Geometry check sheet. Reference: the model listing, model coordinates, mm. A direction names the side the tool comes from. Coordinates: 2 decimals unless noted, no trailing zeros. Write each loop counter-clockwise with the first axis right and the second up, starting at its lowest first coordinate (ties: lowest second). Pieces come first, ordered by that corner, then holes.
from build123d import *

# Parameters (mm, degrees)
F0_R      = 16.129
F1_DEPTH  = 12.7
F2_R      = 22.479
F2_R_2    = 16.129
F3_DEPTH  = 12.7
F5_D      = 3.2639
F5_DEPTH  = 19.05
F5_TIP    = 0.9805744872
F7_DEPTH  = 12.7
F8_R      = 12.7
F9_R      = 7.366
F10_DEPTH = 152.4
F11_R     = 1.27
F13_D     = 3.175
F13_DEPTH = 12.7
F13_TIP   = 0.9538662327
F15_D     = 4.7625
F15_DEPTH = 19.05
F15_TIP   = 1.4307993491
F16_W     = 25.4
F16_H     = 25.5016
F17_DEPTH = 4.7625


with BuildPart() as f1:
    # F0 (on Top) → F1 (new body)
    with BuildSketch(Plane.XY):
        with BuildLine():
            Line((0, 133.35), (0, 0))
            Line((0, 0), (95.25, 0))
            ThreePointArc((95.25, 0), (99.7401280605, 1.8598719395), (101.6, 6.35))
            Line((101.6, 6.35), (101.6, 133.35))
            ThreePointArc((101.6, 133.35), (99.7401280605, 137.8401280605), (95.25, 139.7))
            Line((95.25, 139.7), (6.35, 139.7))
            ThreePointArc((6.35, 139.7), (1.8598719395, 137.8401280605), (0, 133.35))
        make_face()
        with Locations((25.4, 53.975)):
            Circle(F0_R, mode=Mode.SUBTRACT)
    extrude(amount=F1_DEPTH)

    # F2 (on face) → F3 (join)
    with BuildSketch(Plane.XY.offset(12.7)):
        with Locations((25.4, 53.975)):
            Circle(F2_R)
        with Locations((25.4, 53.975)):
            Circle(F2_R_2, mode=Mode.SUBTRACT)
    extrude(amount=F3_DEPTH)

    # F5
    with Locations(Plane.XY.offset(12.7)):
        with Locations((88.265, 127), (88.265, 114.3)):
            Hole(F5_D / 2, depth=F5_DEPTH)
            with Locations((0, 0, -(F5_DEPTH + F5_TIP / 2))):  # 118° drill point
                Cone(0, F5_D / 2, F5_TIP, mode=Mode.SUBTRACT)

    # F6 (on face) → F7 (cut, through all)
    with BuildSketch(Plane.XY.offset(12.7)):
        Polygon((95.25, 0), (0, 28.575), (0, 0), align=None)
        Polygon((0, 139.7), (0, 76.2), (69.85, 139.7), align=None)
    extrude(amount=-F7_DEPTH, mode=Mode.SUBTRACT)

    # F8
    f8_edges = [f1.edges().sort_by_distance(p)[0] for p in [
        (0, 28.575, 6.35),
        (0, 76.2, 6.35),
        (69.85, 139.7, 6.35),
        (95.25, 0, 6.35),
    ]]
    fillet(f8_edges, radius=F8_R)

    # F9 (on Front) → F10 (cut)
    with BuildSketch(Plane.XZ):
        with Locations((76.2, 15.875)):
            Circle(F9_R)
    extrude(amount=-F10_DEPTH, mode=Mode.SUBTRACT)

    # F11
    f11_edges = [f1.edges().sort_by_distance(p)[0] for p in [
        (2.921, 53.975, 25.4),
    ]]
    fillet(f11_edges, radius=F11_R)

    # F13
    with Locations(Plane(origin=(0, 0, 0), x_dir=(0, 1, 0), z_dir=(-1, 0, 0))):
        with Locations((53.975, -18.3411143556)):
            Hole(F13_D / 2, depth=F13_DEPTH)
            with Locations((0, 0, -(F13_DEPTH + F13_TIP / 2))):  # 118° drill point
                Cone(0, F13_D / 2, F13_TIP, mode=Mode.SUBTRACT)

    # F15
    with Locations(Plane.XY.offset(12.7)):
        with Locations((88.9, 101.6), (88.9, 88.9), (63.5, 101.6), (63.5, 88.9), (63.5, 31.75), (63.5, 19.05), (88.9, 19.05), (88.9, 31.75)):
            Hole(F15_D / 2, depth=F15_DEPTH)
            with Locations((0, 0, -(F15_DEPTH + F15_TIP / 2))):  # 118° drill point
                Cone(0, F15_D / 2, F15_TIP, mode=Mode.SUBTRACT)

    # F16 (on face) → F17 (cut)
    with BuildSketch(Plane(origin=(0, 0, 0), x_dir=(1, 0, 0), z_dir=(0, 0, -1))):
        with Locations((88.9, -120.5992)):
            Rectangle(F16_W, F16_H)
    extrude(amount=-F17_DEPTH, mode=Mode.SUBTRACT)


solid = f1.part
1. Draft check along X on faces 4 (the flat face through (22, 70, 25.4)), 5 (the flat face through (47.68, 14.27, 6.44)), 6 (the cylindrical face through (87.62, 90.91, 6.26)). Enter one of: released by +X, released by -X, zero draft, split by the parting line, or undercut.
Computed values:
face 4: zero draft
face 5: released by -X
face 6: undercut
2. Gauge pin test, flat ends, axial feed: pin 1 Ø5.5 at (x, y) = (90.5, 49) entering from +Z; pin 2 Ø2.5 at (y, z) = (53.98, 18.34) entering from -X; pin 3 Ø4 at (x, z) = (91.5, 3.5) entering from -Y. Record the tip position at first contact, or that the pin passes through.
Computed values:
pin 1: stops at z = 12.7
pin 2: stops at x = 41.48
pin 3: stops at y = 2.48
3. Sectioned sample at B-B, the plane x = 25.4. Record the boundary of the cut face in (y, z) (3 decimals), and give its area (3 significant figures).
Computed values:
outline: (20.955, 0) - (37.846, 0) - (37.846, 25.4) - (32.766, 25.4) arc R1.27 ccw to (31.496, 24.13) - (31.496, 12.7) - (20.955, 12.7) - close; (70.104, 0) - (99.291, 0) - (99.291, 12.7) - (76.454, 12.7) - (76.454, 24.13) arc R1.27 ccw to (75.184, 25.4) - (70.104, 25.4) - close
area: 746 mm2
4. Sectioned sample at D-D, the plane y = 123. Record the boundary of the cut face in (x, z) (1 decimal), and give its area (3 significant figures).
Computed values:
outline: (51.5, 0) - (76.2, 0) - (76.2, 4.8) - (101.6, 4.8) - (101.6, 12.7) - (82.8, 12.7) arc R7.4 cw to (69.6, 12.7) - (51.5, 12.7) - close
area: 476 mm2
5. Access from +Z, -Z, +X, -X, +Y, -Y to the whole of each face (thin tool, end or side, straight path). Record for faces 1 (the flat face through (89, 133.35, 2)), 2 (the flat face through (92, 72, 12.7)), 3 (the cylindrical face through (63.81, 103.96, 6.26)).
Computed values:
face 1: -Z, +X
face 2: +Z, +X, +Y, -Y
face 3: +Z, -Z
6. Sectioned sample at A-A, the plane y = 88.9. Record the boundary of the cut face in (x, z) (3 decimals), and give its area (3 significant figures).
Computed values:
outline: (13.97, 0) - (61.119, 0) - (61.119, 12.7) - (13.97, 12.7) - close; (65.881, 0) - (86.519, 0) - (86.519, 12.7) - (82.847, 12.7) arc R7.366 cw to (69.553, 12.7) - (65.881, 12.7) - close; (91.281, 0) - (101.6, 0) - (101.6, 12.7) - (91.281, 12.7) - close
area: 952 mm2
7. Thickness scan on line 1 along Y through (x, z) = (63.5, 4.25) (3 decimals); line 2 along Y through (x, z) = (35.5, 6.75) (3 decimals); line 3 along Z through (x, y) = (50, 60). Record the ranges inside material, lowest first.
Computed values:
line 1: y = 9.525 to 16.669, 21.431 to 29.369, 34.131 to 86.519, 91.281 to 99.219, 103.981 to 133.927
line 2: y = 17.925 to 41.4, 66.55 to 108.473
line 3: z = 0 to 12.7
8. Sectioned sample at C-C, the plane x = 63.5. Record the boundary of the cut face in (y, z) (3 decimals).
Computed values:
outline: (9.525, 0) - (16.669, 0) - (16.669, 12.7) - (9.525, 12.7) - close; (21.431, 0) - (29.369, 0) - (29.369, 12.7) - (21.431, 12.7) - close; (34.131, 0) - (86.519, 0) - (86.519, 12.7) - (34.131, 12.7) - close; (91.281, 0) - (99.219, 0) - (99.219, 12.7) - (91.281, 12.7) - close; (103.981, 0) - (133.927, 0) - (133.927, 12.7) - (103.981, 12.7) - close
